Could you check a few things on this model? Use its own coordinates, in mm. A direction names the side the tool comes from. Round coordinates to 2 decimals unless told otherwise and drop trailing zeros. Write each loop counter-clockwise with the first axis right and the second up, starting at its lowest first coordinate (ties: lowest second). Pieces come first, ordered by that corner, then holes. Notation, with made-up numbers: (45, 16) -> (92, 16) arc R23 cw to (92, 28) -> close; hole circle Ø7 at (41.25, -8). An arc over 180 degrees is marked (long way). One line per question, with ' | ' between items. Start each with the question number.
1. Imagine slicing it at B-B, the plane x = 0. List the corners of the cut face in (y, z) for me.
2. Imagine slicing it at C-C, the plane y = 1.5. List the corners of the cut face in (x, z) for me, and give its area (3 significant figures).
3. For pin 1 Ø6 at (y, z) = (3.5, -146.5) entering from -X; pin 2 Ø2 at (y, z) = (2, -35.5) entering from -X; pin 3 Ø5 at (y, z) = (5, -140) entering from +X; pin 4 Ø9 at (x, z) = (0, 0) entering from +Y (3 decimals), each with a flat end and sliding along its axis, tell me the tip position at first contact or that it passes through.
4. If I drill on line 1 along Z through (x, y) = (0, 7.5); line 2 along X through (y, z) = (6.5, 77); line 3 along X through (y, z) = (6, -71.5), over which ranges is the centre line in solid material (lowest first)? Write a range as [from, to].
5. Imagine slicing it at A-A, the plane z = 0. List the corners of the cut face in (x, y) for me.
6. Imagine slicing it at D-D, the plane z = 82.5. List the corners of the cut face in (x, y) for me, and give its area (3 significant figures).
7. For faces 1 (the flat face through (96.96, 4.93, 73.3)), 2 (the flat face through (-15, 5, -122)), 3 (the cylindrical face through (-147.316, 4.93, 78.445)), which set-ups out of +Z, -Z, +X, -X, +Y, -Y let a thin tool reach every point of the face, with its end or its side?
8. Thinking about a two-plate mould opening in X: for faces 4 (the cylindrical face through (-151.66, 4.93, 87.32)), 5 (the flat face through (15, 5, -121)), 6 (the cylindrical face through (-1.301, 4.93, -159.143)), which applies, released by +X, released by -X, zero draft, split by the parting line, or undercut?
from build123d import *

# Parameters (mm, degrees)
SKETCH_1_R          = 6
EXTRUDE_1_DEPTH     = 10
SKETCH_2_R          = 7.5
CUT_EXTRUDE_1_DEPTH = 11


with BuildPart() as part:
    # 草图1 → 凸台-拉伸1 (new body)
    with BuildSketch(Plane(origin=(0, 0, 0), x_dir=(1, 0, 0), z_dir=(0, 1, 0))):
        with BuildLine():
            Line((158.496688705, -74.187597814), (66.713596412, -21.196604771))
            ThreePointArc((66.713596412, -21.196604771), (60.621778265, 35), (15, 68.373971656))
            Line((15, 68.373971656), (15, 174.355957742))
            ThreePointArc((15, 174.355957742), (0, 175), (-15, 174.355957742))
            Line((-15, 174.355957742), (-15, 68.373971656))
            ThreePointArc((-15, 68.373971656), (-60.621778265, 35), (-66.713596412, -21.196604771))
            Line((-66.713596412, -21.196604771), (-158.496688705, -74.187597814))
            ThreePointArc((-158.496688705, -74.187597814), (-151.554445662, -87.5), (-143.496688705, -100.168359928))
            Line((-143.496688705, -100.168359928), (-51.713596412, -47.177366885))
            ThreePointArc((-51.713596412, -47.177366885), (0, -70), (51.713596412, -47.177366885))
            Line((51.713596412, -47.177366885), (143.496688705, -100.168359928))
            ThreePointArc((143.496688705, -100.168359928), (151.554445662, -87.5), (158.496688705, -74.187597814))
        make_face()
        with Locations((0, 165)):
            Circle(SKETCH_1_R, mode=Mode.SUBTRACT)
        with Locations((142.894191624, -82.5)):
            Circle(SKETCH_1_R, mode=Mode.SUBTRACT)
        with Locations((-142.894191624, -82.5)):
            Circle(SKETCH_1_R, mode=Mode.SUBTRACT)
    extrude(amount=EXTRUDE_1_DEPTH)

    # 草图2 → 切除-拉伸1 (cut, through all)
    with BuildSketch(Plane(origin=(0, 10, 0), x_dir=(1, 0, 0), z_dir=(0, 1, 0))):
        Circle(SKETCH_2_R)
    extrude(amount=-CUT_EXTRUDE_1_DEPTH, mode=Mode.SUBTRACT)


solid = part.part
Geometry results:
1) outline: (0, -175) -> (10, -175) -> (10, -171) -> (0, -171) -> close; (0, -159) -> (10, -159) -> (10, -7.5) -> (0, -7.5) -> close; (0, 7.5) -> (10, 7.5) -> (10, 70) -> (0, 70) -> close
2) outline: (-158.5, 74.19) -> (-66.71, 21.2) arc R70 ccw to (-15, -68.37) -> (-15, -174.36) arc R175 ccw to (15, -174.36) -> (15, -68.37) arc R70 ccw to (66.71, 21.2) -> (158.5, 74.19) arc R175 ccw to (143.5, 100.17) -> (51.71, 47.18) arc R70 ccw to (-51.71, 47.18) -> (-143.5, 100.17) arc R175 ccw to start; hole circle Ø12 at (-142.89, 82.5); hole circle Ø15 at (0, 0); hole circle Ø12 at (0, -165); hole circle Ø12 at (142.89, 82.5) | area: 24,400 mm2
3) pin 1: stops at x = -15 | pin 2: stops at x = -60.91 | pin 3: stops at x = 15 | pin 4: passes through
4) line 1: z = [-175, -171], [-159, -7.5], [7.5, 70] | line 2: x = [-157.15, -145.29], [-140.5, -103.37], [103.37, 140.5], [145.29, 157.15] | line 3: x = [-15, 15]
5) outline: (-70, 0) -> (-7.5, 0) -> (-7.5, 10) -> (-70, 10) -> close; (7.5, 0) -> (70, 0) -> (70, 10) -> (7.5, 10) -> close
6) outline: (-154.33, 0) -> (-148.89, 0) -> (-148.89, 10) -> (-154.33, 10) -> close; (-136.89, 0) -> (-112.89, 0) -> (-112.89, 10) -> (-136.89, 10) -> close; (112.89, 0) -> (136.89, 0) -> (136.89, 10) -> (112.89, 10) -> close; (148.89, 0) -> (154.33, 0) -> (154.33, 10) -> (148.89, 10) -> close | area: 589 mm2
7) face 1: +Z, +Y, -Y | face 2: -Z, -X, +Y, -Y | face 3: +Y, -Y
8) face 4: released by -X | face 5: released by +X | face 6: undercut
